```python
from build123d import *

# Parameters (mm, degrees)
F0_W     = 40
F0_H     = 20
F1_DEPTH = 300
F2_W     = 110
F2_H     = 40
F2_W_2   = 40
F3_DEPTH = 20
F4_R     = 2


with BuildPart() as f1:
    # F0 (on Top) → F1 (new body)
    with BuildSketch(Plane.XY):
        with Locations((-28.588508, 29.951763)):
            Rectangle(F0_W, F0_H)
    extrude(amount=F1_DEPTH)

    # F2 (on face) → F3 (join)
    with BuildSketch(Plane(origin=(0, 39.951763, 0), x_dir=(-1, 0, 0), z_dir=(0, 1, 0))):
        with Locations((103.588508, 280)):
            Rectangle(F2_W, F2_H)
        with Locations((28.588508, 280)):
            Rectangle(F2_W_2, F2_H)
        with Locations((28.588508, 20)):
            Rectangle(F2_W_2, F2_H)
        with Locations((103.588508, 20)):
            Rectangle(F2_W, F2_H)
    extrude(amount=-F3_DEPTH)

    # F4
    f4_edges = [f1.edges().sort_by_distance(p)[0] for p in [
        (-103.588508, 19.951763, 260),
        (-48.588508, 19.951763, 150),
        (-8.588508, 19.951763, 150),
        (-83.588508, 19.951763, 300),
        (-158.588508, 19.951763, 280),
        (-158.588508, 39.951763, 280),
        (-158.588508, 29.951763, 260),
        (-158.588508, 29.951763, 300),
        (-83.588508, 39.951763, 300),
        (-103.588508, 39.951763, 260),
        (-48.588508, 39.951763, 150),
        (-8.588508, 39.951763, 150),
        (-8.588508, 29.951763, 0),
        (-83.588508, 39.951763, 0),
        (-83.588508, 19.951763, 0),
        (-158.588508, 29.951763, 0),
        (-158.588508, 39.951763, 20),
        (-158.588508, 19.951763, 20),
        (-103.588508, 19.951763, 40),
        (-103.588508, 39.951763, 40),
    ]]
    fillet(f4_edges, radius=F4_R)


solid = f1.part
```
Geometry check sheet. Reference: the model listing, model coordinates, mm. A direction names the side the tool comes from. Coordinates: 2 decimals unless noted, no trailing zeros. Order: outer loops, then holes, each group sorted by start corner. A loop starts at its lowest first (then second) coordinate and runs counter-clockwise, first axis right, second up.
Item 1: Section check C-C (z = 247). Enter the section's corners in (x, y).
Item 2: Depth check by flat-ended pin: pin 1 (12 mm diameter, centred on y = 32.5, z = 247, fed in from -X). Enter the tip coordinate at first touch or a pass-through.
Item 3: Section check B-B (y = 35). Enter the section's corners in (x, z), plus the area to 3 significant figures.
Item 4: Mould release check, pull along Z, two halves, no side actions. Record for faces 1 (the flat face through (-84, 30, 300)), 2 (the flat face through (-104, 30, 40)), 3 (the flat face through (-158.589, 30, 280)): released by +Z, released by -Z, zero draft, split by the parting line, or undercut.
Item 5: Scan lines: line 1 along Z through (x, y) = (-102.5, 28.25); line 2 along X through (y, z) = (34, 218); line 3 along Z through (x, y) = (-83, 39.25). Record each from-to range of solid material in increasing order.
Item 6: Tool access check on faces 4 (the flat face through (-48.589, 30, 148)), 5 (the flat face through (-34, 39.952, 152)). Record the directions out of +Z, -Z, +X, -X, +Y, -Y that give a thin tool (end or side, any length) a straight path to the whole face; none if there is none.
Item 7: Section check A-A (x = -116.5). Enter the section's corners in (y, z).
Check sheet entries:
1. outline: (-48.59, 21.95) arc R2 ccw to (-46.59, 19.95) - (-10.59, 19.95) arc R2 ccw to (-8.59, 21.95) - (-8.59, 37.95) arc R2 ccw to (-10.59, 39.95) - (-46.59, 39.95) arc R2 ccw to (-48.59, 37.95) - close
2. pin 1: stops at x = -48.59
3. outline: (-158.59, 2) arc R2 ccw to (-156.59, 0) - (-10.59, 0) arc R2 ccw to (-8.59, 2) - (-8.59, 300) - (-156.59, 300) arc R2 ccw to (-158.59, 298) - (-158.59, 262) arc R2 ccw to (-156.59, 260) - (-48.59, 260) - (-48.59, 40) - (-158.59, 40) - close
3. area: 20,800 mm2
4. face 1: released by +Z
4. face 2: undercut
4. face 3: zero draft
5. line 1: z = 0 to 40, 260 to 300
5. line 2: x = -48.59 to -8.59
5. line 3: z = 0.48 to 39.52, 260.48 to 299.52
6. face 4: -X, +Y, -Y
6. face 5: +Z, -Z, +X, -X, +Y
7. outline: (19.95, 2) arc R2 ccw to (21.95, 0) - (37.95, 0) arc R2 ccw to (39.95, 2) - (39.95, 38) arc R2 ccw to (37.95, 40) - (21.95, 40) arc R2 ccw to (19.95, 38) - close; (19.95, 262) arc R2 ccw to (21.95, 260) - (37.95, 260) arc R2 ccw to (39.95, 262) - (39.95, 298) arc R2 ccw to (37.95, 300) - (21.95, 300) arc R2 ccw to (19.95, 298) - close
